```python
from build123d import *

# Parameters (mm, degrees)
SKETCH1_R             = 6.255
BOTTOM_RING_DEPTH     = 1.66
SKETCH2_R             = 4.755
MAIN_CYLINDER_DEPTH   = 44.41
SKETCH3_R             = 2.57
TOP_CYLINDER_DEPTH    = 52.56
CUTOUT_PT1_DEPTH      = 33.28
CUTOUT_PT2_DEPTH      = 24.44
SKETCH6_R             = 3.47
BOTTOM_HOLE_PT1_DEPTH = 8.82
SKETCH7_R             = 0.905
TOP_HOLE_DEPTH        = 53.56
BOTTOM_HOLE_PT2_DEPTH = 43.23


with BuildPart() as part:
    # Sketch1 → Bottom Ring (new body)
    with BuildSketch(Plane(origin=(0, 0, 0), x_dir=(1, 0, 0), z_dir=(0, 1, 0))):
        Circle(SKETCH1_R)
    extrude(amount=BOTTOM_RING_DEPTH)

    # Sketch2 → Main Cylinder (add)
    with BuildSketch(Plane(origin=(0, 0, 0), x_dir=(1, 0, 0), z_dir=(0, 1, 0))):
        Circle(SKETCH2_R)
    extrude(amount=MAIN_CYLINDER_DEPTH)

    # Sketch3 → Top Cylinder (add)
    with BuildSketch(Plane(origin=(0, 0, 0), x_dir=(1, 0, 0), z_dir=(0, 1, 0))):
        Circle(SKETCH3_R)
    extrude(amount=TOP_CYLINDER_DEPTH)

    # Sketch4 → Cutout pt1 (cut)
    with BuildSketch(Plane(origin=(0, 44.41, 0), x_dir=(1, 0, 0), z_dir=(0, 1, 0))):
        with BuildLine():
            Line((-0.805, -2.605), (-0.805, -4.686363195))
            ThreePointArc((-0.805, -4.686363195), (-2.608092205, -3.97591248), (-3.977939165, -2.605))
            Line((-3.977939165, -2.605), (-0.805, -2.605))
        make_face()
        with BuildLine():
            Line((0.805, -2.605), (0.805, -4.686363195))
            ThreePointArc((0.805, -4.686363195), (2.608092205, -3.97591248), (3.977939165, -2.605))
            Line((3.977939165, -2.605), (0.805, -2.605))
        make_face()
    extrude(amount=-CUTOUT_PT1_DEPTH, mode=Mode.SUBTRACT)

    # Sketch5 → Cutout pt2 (cut)
    with BuildSketch(Plane(origin=(0, 44.41, 0), x_dir=(1, 0, 0), z_dir=(0, 1, 0))):
        with BuildLine():
            Line((-0.805, -2.605), (-0.805, -4.686363195))
            ThreePointArc((-0.805, -4.686363195), (0, -4.755), (0.805, -4.686363195))
            Line((0.805, -4.686363195), (0.805, -2.605))
            Line((0.805, -2.605), (-0.805, -2.605))
        make_face()
    extrude(amount=-CUTOUT_PT2_DEPTH, mode=Mode.SUBTRACT)

    # Sketch6 → Bottom Hole pt1 (cut)
    with BuildSketch(Plane(origin=(0, 0, 0), x_dir=(1, 0, 0), z_dir=(0, 1, 0))):
        Circle(SKETCH6_R)
    extrude(amount=BOTTOM_HOLE_PT1_DEPTH, mode=Mode.SUBTRACT)

    # Sketch7 → Top Hole (cut, through all)
    with BuildSketch(Plane(origin=(0, 52.56, 0), x_dir=(1, 0, 0), z_dir=(0, 1, 0))):
        Circle(SKETCH7_R)
    extrude(amount=-TOP_HOLE_DEPTH, mode=Mode.SUBTRACT)

    # Sketch8 → Bottom Hole pt2 (cut)
    with BuildSketch(Plane(origin=(0, 0, 0), x_dir=(1, 0, 0), z_dir=(0, 1, 0))):
        with BuildLine():
            Line((-3.33456144, -0.96), (3.33456144, -0.96))
            ThreePointArc((3.33456144, -0.96), (0, 3.47), (-3.33456144, -0.96))
        make_face()
    extrude(amount=BOTTOM_HOLE_PT2_DEPTH, mode=Mode.SUBTRACT)


solid = part.part
```
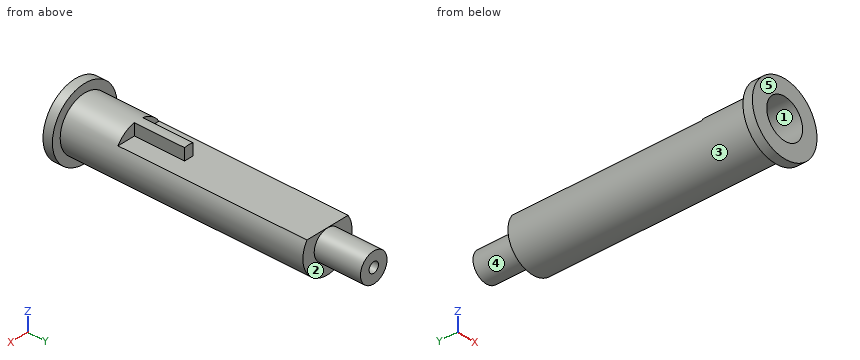
Check sheet for the modelled part. Datum: model origin and axes. Units: mm. Face numbers are marked on the shaded views. A direction names the side the tool comes from. Round coordinates to 2 decimals unless told otherwise and drop trailing zeros. Order: outer loops, then holes, each group sorted by start corner. A loop starts at its lowest first (then second) coordinate and runs counter-clockwise, first axis right, second up. Notation, with made-up numbers: M 24,31 L 78,31 A24 ccw 78,52 Z; hole C 59.25,52 d3. An arc over 180 degrees is marked long. Answer in a Markdown table with one row per item.
(1) Draft check along Z on the marked faces 1, 2 and 3. Enter one of: +Z half, -Z half, draft (parallel to the pull), parting line (faces both ways), or undercut.
Findings:
| item | result |
|---|---|
| face 1 | undercut |
| face 2 | draft |
| face 3 | parting line |
(2) Section check A-A on x = 0. Record the boundary of the cut face in (y, z) (3 decimals).
Findings:
| item | result |
|---|---|
| outline | M 0,-6.255 L 1.66,-6.255 L 1.66,-4.755 L 44.41,-4.755 L 44.41,-2.57 L 52.56,-2.57 L 52.56,-0.905 L 43.23,-0.905 L 43.23,-3.47 L 0,-3.47 Z; M 0,3.47 L 8.82,3.47 L 8.82,0.96 L 43.23,0.96 L 43.23,0.905 L 52.56,0.905 L 52.56,2.57 L 44.41,2.57 L 44.41,2.605 L 19.97,2.605 L 19.97,4.755 L 1.66,4.755 L 1.66,6.255 L 0,6.255 Z |
(3) Gauge pin test, flat ends, axial feed: pin 1 (1.5 mm diameter, centred on x = 3, z = -1.5, fed in from -Y); pin 2 (1.5 mm diameter, centred on y = 17.5, z = -1.5, fed in from -X); pin 3 (0.6 mm diameter, centred on x = -2, z = 3.5, fed in from +Y); pin 4 (2 mm diameter, centred on x = -1, y = 18.5, fed in from -Z) (3 decimals). Record the tip position at first contact, or that the pin passes through.
Findings:
| item | result |
|---|---|
| pin 1 | stops at y = 0 |
| pin 2 | stops at x = -4.7 |
| pin 3 | stops at y = 11.13 |
| pin 4 | stops at z = -4.755 |
(4) Set-up check for the marked faces 4 and 5: record each of +Z, -Z, +X, -X, +Y, -Y from which the full face is reachable in a straight line by a thin tool's end or side.
Findings:
| item | result |
|---|---|
| face 4 | +Y |
| face 5 | +Z, -Z, +X, -X, -Y |
(5) Material ranges on line 1 along X through (y, z) = (49, 0) (3 decimals); line 2 along Z through (x, y) = (0, 24) (3 decimals), recorded low to high. Write a range as from..to.
Findings:
| item | result |
|---|---|
| line 1 | x = -2.57..-0.905, 0.905..2.57 |
| line 2 | z = -4.755..-3.47, 0.96..2.605 |
(6) Section check C-C on x = 2. Record the boundary of the cut face in (y, z) (3 decimals).
Findings:
| item | result |
|---|---|
| outline | M 0,-5.927 L 1.66,-5.927 L 1.66,-4.314 L 44.41,-4.314 L 44.41,-1.614 L 52.56,-1.614 L 52.56,1.614 L 44.41,1.614 L 44.41,2.605 L 11.13,2.605 L 11.13,4.314 L 1.66,4.314 L 1.66,5.927 L 0,5.927 L 0,2.836 L 8.82,2.836 L 8.82,0.96 L 43.23,0.96 L 43.23,-2.836 L 0,-2.836 Z |
(7) Section check B-B on y = 33.5. Record the boundary of the cut face in (x, z) (3 decimals).
Findings:
| item | result |
|---|---|
| outline | M -3.978,2.605 A4.755 ccw long 3.978,2.605 Z; hole M -3.335,0.96 A3.47 ccw long 3.335,0.96 Z |
(8) Section check D-D on y = 48.5. Record the boundary of the cut face in (x, z) (3 decimals), plus the area to 3 significant figures.
Findings:
| item | result |
|---|---|
| outline | C 0,0 d5.14; hole C 0,0 d1.81 |
| area | 18.2 mm^2 |
